Geometry: final body of the model. Coordinates: model frame, mm. A direction names the side the tool comes from. Give positions to 0.01 mm unless a question says otherwise; leave off trailing zeros.
```python
from build123d import *

# Parameters (mm, degrees)
BOSS_EXTRUDE1_DEPTH     = 6.752040791
BOSS_EXTRUDE1_TAPER     = 31.717474411
SKETCH3_R               = 1
CUT_EXTRUDE1_DEPTH      = 2
CIRPATTERN1_COUNT       = 5
MIRROR3_COPY_1_SKETCH_R = 1
MIRROR3_COPY_1_DEPTH    = 2
MIRROR3_COPY_2_SKETCH_R = 1
MIRROR3_COPY_2_DEPTH    = 2
MIRROR3_COPY_3_SKETCH_R = 1
MIRROR3_COPY_3_DEPTH    = 2
MIRROR3_COPY_4_SKETCH_R = 1
MIRROR3_COPY_4_DEPTH    = 2
MIRROR5_COPY_1_SKETCH_R = 1
MIRROR5_COPY_1_DEPTH    = 2
MIRROR5_COPY_2_SKETCH_R = 1
MIRROR5_COPY_2_DEPTH    = 2
MIRROR5_COPY_3_SKETCH_R = 1
MIRROR5_COPY_3_DEPTH    = 2
MIRROR5_COPY_4_SKETCH_R = 1
MIRROR5_COPY_4_DEPTH    = 2


with BuildPart() as part:
    # Sketch1 → Boss-Extrude1 (new body)
    with BuildSketch(Plane(origin=(0, 0, 0), x_dir=(1, 0, 0), z_dir=(0, 1, 0))):
        Polygon((0, 10.803265266), (-10.274515829, 3.338392562), (-6.35, -8.740025195), (6.35, -8.740025195), (10.274515829, 3.338392562), align=None)
    boss_extrude1 = extrude(amount=BOSS_EXTRUDE1_DEPTH, taper=BOSS_EXTRUDE1_TAPER)

    # Sketch3 → Cut-Extrude1 (cut)
    with BuildSketch(Plane(origin=(0, 3.908658092, 6.324341644), x_dir=(1, 0, 0), z_dir=(0, 0.525731112, 0.850650808))):
        with Locations((-2, -0.626153166)):
            Circle(SKETCH3_R)
        with Locations((2, -0.626153166)):
            Circle(SKETCH3_R)
    cut_extrude1 = extrude(amount=-CUT_EXTRUDE1_DEPTH, mode=Mode.SUBTRACT)

    # CirPattern1: Cut-Extrude1 ×5 about axis
    cirpattern1_axis = Axis((0, 0, 0), (0, 1, 0))
    for i in range(1, CIRPATTERN1_COUNT):
        add(cut_extrude1.rotate(cirpattern1_axis, i * 360 / CIRPATTERN1_COUNT), mode=Mode.SUBTRACT)

    # Mirror3: Boss-Extrude1, Cut-Extrude1 across plane
    add(boss_extrude1.mirror(Plane(origin=(-6.35, 0, 8.740025195), x_dir=(0, -0.850650808, 0.525731112), z_dir=(0, 0.525731112, 0.850650808))))
    add(cut_extrude1.mirror(Plane(origin=(-6.35, 0, 8.740025195), x_dir=(0, -0.850650808, 0.525731112), z_dir=(0, 0.525731112, 0.850650808))), mode=Mode.SUBTRACT)

    # Mirror3 copy 1 sketch → Mirror3 copy 1 (cut)
    with BuildSketch(Plane(origin=(6.014806331, 7.817316184, 8.27867069), x_dir=(0.309016994, 0.850650808, 0.425325404), z_dir=(0.809016994, 0, -0.587785252))):
        with Locations((-2, 0.626153166)):
            Circle(MIRROR3_COPY_1_SKETCH_R)
        with Locations((2, 0.626153166)):
            Circle(MIRROR3_COPY_1_SKETCH_R)
    extrude(amount=-MIRROR3_COPY_1_DEPTH, mode=Mode.SUBTRACT)

    # Mirror3 copy 2 sketch → Mirror3 copy 2 (cut)
    with BuildSketch(Plane(origin=(3.717354749, 14.141657828, 11.440841512), x_dir=(-0.809016994, 0.525731112, 0.262865556), z_dir=(0.5, 0.850650808, -0.162459848))):
        with Locations((-2, 0.626153166)):
            Circle(MIRROR3_COPY_2_SKETCH_R)
        with Locations((2, 0.626153166)):
            Circle(MIRROR3_COPY_2_SKETCH_R)
    extrude(amount=-MIRROR3_COPY_2_DEPTH, mode=Mode.SUBTRACT)

    # Mirror3 copy 3 sketch → Mirror3 copy 3 (cut)
    with BuildSketch(Plane(origin=(-3.717354749, 14.141657828, 11.440841512), x_dir=(-0.809016994, -0.525731112, -0.262865556), z_dir=(-0.5, 0.850650808, -0.162459848))):
        with Locations((-2, 0.626153166)):
            Circle(MIRROR3_COPY_3_SKETCH_R)
        with Locations((2, 0.626153166)):
            Circle(MIRROR3_COPY_3_SKETCH_R)
    extrude(amount=-MIRROR3_COPY_3_DEPTH, mode=Mode.SUBTRACT)

    # Mirror3 copy 4 sketch → Mirror3 copy 4 (cut)
    with BuildSketch(Plane(origin=(-6.014806331, 7.817316184, 8.27867069), x_dir=(0.309016994, -0.850650808, -0.425325404), z_dir=(-0.809016994, 0, -0.587785252))):
        with Locations((-2, 0.626153166)):
            Circle(MIRROR3_COPY_4_SKETCH_R)
        with Locations((2, 0.626153166)):
            Circle(MIRROR3_COPY_4_SKETCH_R)
    extrude(amount=-MIRROR3_COPY_4_DEPTH, mode=Mode.SUBTRACT)

    # Mirror5: Boss-Extrude1, Cut-Extrude1 across plane
    add(boss_extrude1.mirror(Plane(origin=(10.274515829, 0, -3.338392562), x_dir=(0.47426801, 0.498674897, 0.725529601), z_dir=(0.5, 0.525731112, -0.68819096))))
    add(cut_extrude1.mirror(Plane(origin=(10.274515829, 0, -3.338392562), x_dir=(0.47426801, 0.498674897, 0.725529601), z_dir=(0.5, 0.525731112, -0.68819096))), mode=Mode.SUBTRACT)

    # Mirror5 copy 1 sketch → Mirror5 copy 1 (cut)
    with BuildSketch(Plane(origin=(9.73216108, 7.817316184, -3.162170822), x_dir=(-0.5, -0.850650808, 0.162459848), z_dir=(0.309016994, 0, 0.951056516))):
        with Locations((-2, 0.626153166)):
            Circle(MIRROR5_COPY_1_SKETCH_R)
        with Locations((2, 0.626153166)):
            Circle(MIRROR5_COPY_1_SKETCH_R)
    extrude(amount=-MIRROR5_COPY_1_DEPTH, mode=Mode.SUBTRACT)

    # Mirror5 copy 2 sketch → Mirror5 copy 2 (cut)
    with BuildSketch(Plane(origin=(3.717354749, 3.908658092, -5.116499868), x_dir=(-0.809016994, 0, -0.587785252), z_dir=(-0.5, -0.525731112, 0.68819096))):
        with Locations((-2, 0.626153166)):
            Circle(MIRROR5_COPY_2_SKETCH_R)
        with Locations((2, 0.626153166)):
            Circle(MIRROR5_COPY_2_SKETCH_R)
    extrude(amount=-MIRROR5_COPY_2_DEPTH, mode=Mode.SUBTRACT)

    # Mirror5 copy 3 sketch → Mirror5 copy 3 (cut)
    with BuildSketch(Plane(origin=(0, 7.817316184, -10.232999736), x_dir=(0, 0.850650808, -0.525731112), z_dir=(-1, 0, 0))):
        with Locations((-2, 0.626153166)):
            Circle(MIRROR5_COPY_3_SKETCH_R)
        with Locations((2, 0.626153166)):
            Circle(MIRROR5_COPY_3_SKETCH_R)
    extrude(amount=-MIRROR5_COPY_3_DEPTH, mode=Mode.SUBTRACT)

    # Mirror5 copy 4 sketch → Mirror5 copy 4 (cut)
    with BuildSketch(Plane(origin=(3.717354749, 14.141657828, -11.440841512), x_dir=(0.809016994, 0.525731112, 0.262865556), z_dir=(-0.5, 0.850650808, -0.162459848))):
        with Locations((-2, 0.626153166)):
            Circle(MIRROR5_COPY_4_SKETCH_R)
        with Locations((2, 0.626153166)):
            Circle(MIRROR5_COPY_4_SKETCH_R)
    extrude(amount=-MIRROR5_COPY_4_DEPTH, mode=Mode.SUBTRACT)


solid = part.part
```
Q1. Reachability of faces 4 (the face through (0.986, 8.557, -12.592)), 5 (the face through (4.5, 11.4, 11.8)) from +Z, -Z, +X, -X, +Y, -Y: full face, straight path, thin tool, end or side. Return the list, or none.
Q2. Mould query, pull axis Y, two halves, no side actions, for faces 1 (the face through (-0.807, 8.187, 12.834)), 2 (the face through (0.986, 5.801, -10.714)), 3 (the face through (-5.715, 3.113, -2.84)). Classes: +Y half, -Y half, draft (parallel to the pull), parting line (faces both ways), or undercut.
Q3. Pin query (flat end, axial travel): pin 1 Ø1.6 at (y, z) = (9.19, -11.82) entering from +X; pin 2 Ø1.5 at (y, z) = (9, 0) entering from -X; pin 3 Ø6 at (x, z) = (9.5, -13) entering from +Y; pin 4 Ø3 at (x, z) = (2.5, -1.5) entering from +Y. Return the tip coordinate at first contact, or that it passes through.
Q4. Material intervals for probe 1 along Z at (x, y) = (5, 2); probe 2 along Y at (x, z) = (3, 1); probe 3 along Z at (x, y) = (8, 9.25), sorted ascending.
Resolved:
1. face 4: -X
1. face 5: none
2. face 1: -Y half
2. face 2: undercut
2. face 3: undercut
3. pin 1: stops at x = 7.71
3. pin 2: passes through
3. pin 3: stops at y = 17.48
3. pin 4: stops at y = 6.75
4. probe 1: z = -8.41 to -4.05, -2.74 to 2.93, 4.26 to 9.74
4. probe 2: y = 0 to 6.75
4. probe 3: z = -10.71 to -2.6, 11.01 to 13.37
